Solid Edge part; units mm, degrees
sketch "Sketch1" plane through (0, 0, 0) normal (0, -1, 0) x (1, 0, 0)
  line L0 (-51.5, 15) -> (51.5, 15)
  line L1 (51.5, 15) -> (51.5, -15)
  line L2 (51.5, -15) -> (-51.5, -15)
  line L3 (-51.5, -15) -> (-51.5, 15)
  dimension "D1" = 51.5
  dimension "D2" = 51.5
extrude "Protrusion1" add sketch "Sketch1" along normal mid plane 6
hole "Bohrung_1" at (47.5, -3, 10) direction (0, 1, 0) diameter 3.5 end through all
hole "Hole1" at (47.5, -3, -10) direction (0, 1, 0) diameter 3.5 end through all
hole "Hole2" at (-47.5, -3, -10) direction (0, 1, 0) diameter 3.5 end through all
hole "Hole3" at (-47.5, -3, 10) direction (0, 1, 0) diameter 3.5 end through all
sketch "Sketch2" plane through (0, -3, 0) normal (0, -1, 0) x (1, 0, 0)
  line L0 (26.5, 15) -> (38.5, 15)
  line L1 (38.5, 15) -> (38.5, -6)
  line L2 (38.5, -6) -> (26.5, -6)
  line L3 (26.5, -6) -> (26.5, 15)
  dimension "D1" = 26.5
  dimension "D2" = 38.5
extrude "Ausschnitt_1" cut sketch "Sketch2" against normal blind 168.275
hole "Bohrung_5" at (22.5, -3, 0) direction (0, 1, 0) diameter 3.5 depth 2
hole "Hole4" at (42.5, -3, 0) direction (0, 1, 0) diameter 3.5 depth 2
hole "Bohrung_9" at (-34.5, -3, 0) direction (0, 1, 0) diameter 6.35 depth 1
hole "Hole5" at (-13.5, -3, 0) direction (0, 1, 0) diameter 6.35 depth 1
sketch "Sketch3" plane through (0, -3, 0) normal (0, -1, 0) x (1, 0, 0)
  line L0 (-0.9853, 0) -> (7.5, -8.4853)
  line L1 (7.5, -8.4853) -> (30.9853, 15)
  line L2 (14.0147, 15) -> (30.9853, 15)
  line L3 (-0.9853, 0) -> (14.0147, 15)
  dimension "D1" = 0.9853
extrude "Ausschnitt_5" cut sketch "Sketch3" against normal blind 285.75
hole "Bohrung_11" at (14.5711, -3, -7.0711) direction (0, 1, 0) diameter 3.5 depth 2
hole "Hole6" at (0.4289, -3, 7.0711) direction (0, 1, 0) diameter 3.5 depth 2
hole "Bohrung_13" at (-34.5, 3, 0) direction (0, -1, 0) diameter 10.5 depth 5
hole "Hole7" at (-13.5, 3, 0) direction (0, -1, 0) diameter 10.5 depth 5
hole "Bohrung_15" at (14.5711, 3, -7.0711) direction (0, -1, 0) diameter 6 depth 4
hole "Hole8" at (0.4289, 3, 7.0711) direction (0, -1, 0) diameter 6 depth 4
hole "Hole9" at (22.5, 3, 0) direction (0, -1, 0) diameter 6 depth 4
hole "Hole10" at (42.5, 3, 0) direction (0, -1, 0) diameter 6 depth 4
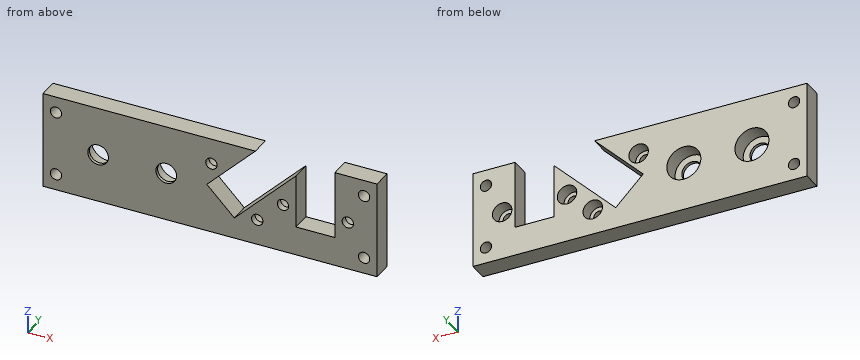
Could you check a few things on this model? Use its own coordinates, in mm. Round coordinates to 2 decimals unless told otherwise and drop trailing zeros. Loops run counter-clockwise (first coordinate to the right, second up) from the corner with the lowest first, then second, coordinate; pieces in that order, holes last. Notation, with made-up numbers: (10, 56.25) -> (69, 56.25) arc R17 cw to (69, 60.25) -> close; hole circle Ø11 at (58, 67.25). An arc over 180 degrees is marked (long way). One line per question, with ' | ' between items.
(1) If we section it at D-D on x = -13.5: List the corners of the cut face in (y, z) for me (3 decimals), and give its area (3 significant figures).
Model answer:
outline: (-3, -15) -> (3, -15) -> (3, -5.25) -> (-2, -5.25) -> (-2, -3.175) -> (-3, -3.175) -> close; (-3, 3.175) -> (-2, 3.175) -> (-2, 5.25) -> (3, 5.25) -> (3, 15) -> (-3, 15) -> close | area: 121 mm^2
(2) If I drill on probe 1 along Z at (x, y) = (-47.5, 0.05); probe 2 along Z at (x, y) = (-13.5, 1.6); probe 3 along X at (y, z) = (-1.55, -4.5), over which ranges is the centre line in solid material (lowest first)?
Model answer:
probe 1: z = -15 to -11.75, -8.25 to 8.25, 11.75 to 15 | probe 2: z = -15 to -5.25, 5.25 to 15 | probe 3: x = -51.5 to -37.2, -31.8 to -16.2, -10.8 to 3.51, 11.49 to 26.5, 38.5 to 51.5
(3) If we section it at A-A on x = 42.5: List the corners of the cut face in (y, z) for me, and give its area (3 significant figures).
Model answer:
outline: (-3, -15) -> (3, -15) -> (3, -3) -> (-1, -3) -> (-1, -1.75) -> (-3, -1.75) -> close; (-3, 1.75) -> (-1, 1.75) -> (-1, 3) -> (3, 3) -> (3, 15) -> (-3, 15) -> close | area: 149 mm^2
(4) For pin 1 Ø3 at (x, y) = (33, -1.5) entering from +Z; pin 2 Ø5 at (x, z) = (-13.5, 1.5) entering from +Y, each with a flat end and sliding along its axis, tell me the tip position at first contact or that it passes through.
Model answer:
pin 1: stops at z = -6 | pin 2: stops at y = -2
(5) If we section it at C-C on y = 1.3: Count the separate pieces of the cut face and the enclosed holes in it, and give its area (3 significant figures).
Model answer:
separate pieces: 1 | enclosed holes: 10 | area: 2,200 mm^2
(6) If we section it at B-B on x = -47.5: List the corners of the cut face in (y, z) for me, and give its area (3 significant figures).
Model answer:
outline: (-3, -15) -> (3, -15) -> (3, -11.75) -> (-3, -11.75) -> close; (-3, -8.25) -> (3, -8.25) -> (3, 8.25) -> (-3, 8.25) -> close; (-3, 11.75) -> (3, 11.75) -> (3, 15) -> (-3, 15) -> close | area: 138 mm^2
